The listing builds one solid part. Answer for the finished solid, in the listing's coordinates (mm). Face numbers are marked on the shaded views. A direction names the side the tool comes from. Give positions to 0.01 mm unless a question says otherwise; leave off trailing zeros. Write each loop counter-clockwise with the first axis right and the second up, starting at its lowest first coordinate (ties: lowest second). Pieces come first, ordered by that corner, then holes. Notation, with made-up numbers: (5, 45) -> (42, 45) arc R14 ccw to (42, 69) -> close; hole circle Ø11 at (-9.75, -7). An arc over 180 degrees is marked (long way). Put each result on its own line as item: value. Start each with the question number.
1) For a pull along X with two mould halves and no side action, classify the marked faces 1, 2 and 3 as released by +X, released by -X, zero draft, split by the parting line, or undercut.
2) For the marked faces 4, 5 and 6, determine the directions among +Z, -Z, +X, -X, +Y, -Y from which every point of the face is accessible in a straight line to the end or side of a thin tool.
3) Flat-ended cylindrical pins translate along their axes: pin 1 Ø6 at (x, y) = (8, 9.5) entering from +Z; pin 2 Ø6 at (x, z) = (-10.5, -39.5) entering from -Y; pin 3 Ø0.5 at (x, z) = (17.5, -27.5) entering from +Y; pin 4 Ø1 at (y, z) = (-5, -33) entering from -X. Find the tip coordinate at first contact, or state that the pin passes through.
4) Find the intervals of material crossed by line 1 along X through (y, z) = (11, -28.75); line 2 along Z through (x, y) = (7.5, -15.5); line 3 along Z through (x, y) = (-4.5, -20.5), in increasing order. Write a range as from..to.
5) A cutting plane is placed at A-A (z = -36.75). Write down the section's boundary in (x, y), then the cut area to 3 significant figures.
from build123d import *

# Parameters (mm, degrees)
CYLINDER101_R               = 0.8
CYLINDER101_DEPTH           = 5
BOX013_W                    = 2
BOX013_H                    = 5.5
BOX013_DEPTH                = 5
BOX012_W                    = 0.75
BOX012_H                    = 8
BOX012_DEPTH                = 5
CYLINDER100_R               = 3
CYLINDER100_DEPTH           = 5
CUT064_PLACEMENT_ANGLE      = 120
CYLINDER104_R               = 0.8
CYLINDER104_DEPTH           = 5
CUT067_PLACEMENT_ANGLE      = 60
CYLINDER102_R               = 0.8
CYLINDER102_DEPTH           = 5
CUT065_PLACEMENT_ANGLE      = 180
CYLINDER106_R               = 0.8
CYLINDER106_DEPTH           = 5
CYLINDER103_R               = 0.8
CYLINDER103_DEPTH           = 5
CUT066_PLACEMENT_ANGLE      = 240
CYLINDER098_R               = 0.8
CYLINDER098_DEPTH           = 5
CUT063_PLACEMENT_ANGLE      = 60
CYLINDER007_R               = 19.25
CYLINDER007_DEPTH           = 5
CYLINDER018_R               = 22.5
CYLINDER018_DEPTH           = 0.5
CYLINDER070_R               = 20
CYLINDER070_DEPTH           = 5
CYLINDER006_R               = 18.5
CYLINDER006_DEPTH           = 20
CYLINDER002_R               = 22.1
CYLINDER002_DEPTH           = 17
CYLINDER001_R               = 23.5
CYLINDER001_DEPTH           = 17
CYLINDER_R                  = 23.5
CYLINDER_DEPTH              = 20
CYLINDER003_R               = 22
CYLINDER003_DEPTH           = 17
CYLINDER004_R               = 23.5
CYLINDER004_DEPTH           = 10
CUT060_PLACEMENT_ANGLE      = 180
FUSION050_PLACEMENT_ANGLE   = 180
CYLINDER073_R               = 1
CYLINDER073_DEPTH           = 10
CYLINDER073_PLACEMENT_ANGLE = 120
CYLINDER075_R               = 1
CYLINDER075_DEPTH           = 10
CYLINDER075_PLACEMENT_ANGLE = 240
CYLINDER072_R               = 1
CYLINDER072_DEPTH           = 10
CYLINDER072_PLACEMENT_ANGLE = 60
CYLINDER074_R               = 1
CYLINDER074_DEPTH           = 10
CYLINDER076_R               = 1
CYLINDER076_DEPTH           = 10
CYLINDER076_PLACEMENT_ANGLE = 60
CYLINDER071_R               = 1
CYLINDER071_DEPTH           = 10
FUSION030_PLACEMENT_ANGLE   = 30


with BuildPart() as cylinder101:
    # Cylinder101 → Cylinder101 (new body)
    with BuildSketch(Plane(origin=(15.5, 0, 15), x_dir=(1, 0, 0), z_dir=(0, 0, 1))):
        Circle(CYLINDER101_R)
    extrude(amount=CYLINDER101_DEPTH)


with BuildPart() as cube013:
    # Box013 → Box013 (new body)
    with BuildSketch(Plane(origin=(16.5, -2.75, 15), x_dir=(1, 0, 0), z_dir=(0, 0, 1))):
        with Locations((1, 2.75)):
            Rectangle(BOX013_W, BOX013_H)
    extrude(amount=BOX013_DEPTH)


with BuildPart() as cube012:
    # Box012 → Box012 (new body)
    with BuildSketch(Plane(origin=(18.2, -4, 15), x_dir=(1, 0, 0), z_dir=(0, 0, 1))):
        with Locations((0.375, 4)):
            Rectangle(BOX012_W, BOX012_H)
    extrude(amount=BOX012_DEPTH)


with BuildPart() as cylinder100:
    # Cylinder100 → Cylinder100 (new body)
    with BuildSketch(Plane(origin=(15.5, 0, 15), x_dir=(1, 0, 0), z_dir=(0, 0, 1))):
        Circle(CYLINDER100_R)
    extrude(amount=CYLINDER100_DEPTH)


with BuildPart() as cut064:
    # Fusion043 base: copy of Cylinder100
    add(cylinder100.part)

    # Fusion043: union Cube013, Cube012
    add(cube013.part)
    add(cube012.part)

    # Cut064: cut Cylinder101
    add(cylinder101.part, mode=Mode.SUBTRACT)


with BuildPart() as cut064_1:
    # Cut064 placement: moved
    add(cut064.part.moved(Location((0, 0, 9))).rotate(Axis((0, 0, 9), (0, 0, 1)), CUT064_PLACEMENT_ANGLE))


with BuildPart() as cylinder104:
    # Cylinder104 → Cylinder104 (new body)
    with BuildSketch(Plane(origin=(15.5, 0, 15), x_dir=(1, 0, 0), z_dir=(0, 0, 1))):
        Circle(CYLINDER104_R)
    extrude(amount=CYLINDER104_DEPTH)


with BuildPart() as cut067:
    # Fusion046 base: copy of Cylinder100
    add(cylinder100.part)

    # Fusion046: union Cube013, Cube012
    add(cube013.part)
    add(cube012.part)

    # Cut067: cut Cylinder104
    add(cylinder104.part, mode=Mode.SUBTRACT)


with BuildPart() as cut067_1:
    # Cut067 placement: moved
    add(cut067.part.moved(Location((0, 0, 9))).rotate(Axis((0, 0, 9), (0, 0, -1)), CUT067_PLACEMENT_ANGLE))


with BuildPart() as cylinder102:
    # Cylinder102 → Cylinder102 (new body)
    with BuildSketch(Plane(origin=(15.5, 0, 15), x_dir=(1, 0, 0), z_dir=(0, 0, 1))):
        Circle(CYLINDER102_R)
    extrude(amount=CYLINDER102_DEPTH)


with BuildPart() as cut065:
    # Fusion044 base: copy of Cylinder100
    add(cylinder100.part)

    # Fusion044: union Cube013, Cube012
    add(cube013.part)
    add(cube012.part)

    # Cut065: cut Cylinder102
    add(cylinder102.part, mode=Mode.SUBTRACT)


with BuildPart() as cut065_1:
    # Cut065 placement: moved
    add(cut065.part.moved(Location((0, 0, 9))).rotate(Axis((0, 0, 9), (0, 0, 1)), CUT065_PLACEMENT_ANGLE))


with BuildPart() as cylinder106:
    # Cylinder106 → Cylinder106 (new body)
    with BuildSketch(Plane(origin=(15.5, 0, 15), x_dir=(1, 0, 0), z_dir=(0, 0, 1))):
        Circle(CYLINDER106_R)
    extrude(amount=CYLINDER106_DEPTH)


with BuildPart() as cut069:
    # Fusion048 base: copy of Cylinder100
    add(cylinder100.part)

    # Fusion048: union Cube013, Cube012
    add(cube013.part)
    add(cube012.part)

    # Cut069: cut Cylinder106
    add(cylinder106.part, mode=Mode.SUBTRACT)


with BuildPart() as cut069_1:
    # Cut069 placement: moved
    add(cut069.part.moved(Location((0, 0, 9))))


with BuildPart() as cylinder103:
    # Cylinder103 → Cylinder103 (new body)
    with BuildSketch(Plane(origin=(15.5, 0, 15), x_dir=(1, 0, 0), z_dir=(0, 0, 1))):
        Circle(CYLINDER103_R)
    extrude(amount=CYLINDER103_DEPTH)


with BuildPart() as cut066:
    # Fusion045 base: copy of Cylinder100
    add(cylinder100.part)

    # Fusion045: union Cube013, Cube012
    add(cube013.part)
    add(cube012.part)

    # Cut066: cut Cylinder103
    add(cylinder103.part, mode=Mode.SUBTRACT)


with BuildPart() as cut066_1:
    # Cut066 placement: moved
    add(cut066.part.moved(Location((0, 0, 9))).rotate(Axis((0, 0, 9), (0, 0, 1)), CUT066_PLACEMENT_ANGLE))


with BuildPart() as cylinder098:
    # Cylinder098 → Cylinder098 (new body)
    with BuildSketch(Plane(origin=(15.5, 0, 15), x_dir=(1, 0, 0), z_dir=(0, 0, 1))):
        Circle(CYLINDER098_R)
    extrude(amount=CYLINDER098_DEPTH)


with BuildPart() as fusion049:
    # Fusion042 base: copy of Cylinder100
    add(cylinder100.part)

    # Fusion042: union Cube013, Cube012
    add(cube013.part)
    add(cube012.part)

    # Cut063: cut Cylinder098
    add(cylinder098.part, mode=Mode.SUBTRACT)


with BuildPart() as fusion049_1:
    # Cut063 placement: moved
    add(fusion049.part.moved(Location((0, 0, 9))).rotate(Axis((0, 0, 9), (0, 0, 1)), CUT063_PLACEMENT_ANGLE))

    # Fusion049: union Cut064, Cut067, Cut065, Cut069, Cut066
    add(cut064_1.part)
    add(cut067_1.part)
    add(cut065_1.part)
    add(cut069_1.part)
    add(cut066_1.part)


with BuildPart() as cylinder007:
    # Cylinder007 → Cylinder007 (new body)
    with BuildSketch(Plane.XY.offset(5)):
        Circle(CYLINDER007_R)
    extrude(amount=CYLINDER007_DEPTH)


with BuildPart() as cone:
    # Cone → Cone (revolve)
    with BuildSketch(Plane(origin=(0, 0, 5), x_dir=(1, 0, 0), z_dir=(0, -1, 0))):
        Polygon((0, 0), (20, 0), (12, 6), (0, 6), align=None)
    revolve(axis=Axis((0, 0, 5), (0, 0, 1)))


with BuildPart() as cylinder018:
    # Cylinder018 → Cylinder018 (new body)
    with BuildSketch(Plane.XY):
        Circle(CYLINDER018_R)
    extrude(amount=CYLINDER018_DEPTH)


with BuildPart() as cylinder070:
    # Cylinder070 → Cylinder070 (new body)
    with BuildSketch(Plane.XY):
        Circle(CYLINDER070_R)
    extrude(amount=CYLINDER070_DEPTH)


with BuildPart() as cylinder006:
    # Cylinder006 → Cylinder006 (new body)
    with BuildSketch(Plane.XY):
        Circle(CYLINDER006_R)
    extrude(amount=CYLINDER006_DEPTH)


with BuildPart() as cylinder002:
    # Cylinder002 → Cylinder002 (new body)
    with BuildSketch(Plane.XY):
        Circle(CYLINDER002_R)
    extrude(amount=CYLINDER002_DEPTH)


with BuildPart() as cut:
    # Cylinder001 → Cylinder001 (new body)
    with BuildSketch(Plane.XY):
        Circle(CYLINDER001_R)
    extrude(amount=CYLINDER001_DEPTH)

    # Cut: cut Cylinder002
    add(cylinder002.part, mode=Mode.SUBTRACT)


with BuildPart() as cut_1:
    # Cut placement: moved
    add(cut.part.moved(Location((0, 0, 1.5))))


with BuildPart() as cut001:
    # Cylinder → Cylinder (new body)
    with BuildSketch(Plane.XY):
        Circle(CYLINDER_R)
    extrude(amount=CYLINDER_DEPTH)

    # Cut001: cut Cut
    add(cut_1.part, mode=Mode.SUBTRACT)


with BuildPart() as cylinder003:
    # Cylinder003 → Cylinder003 (new body)
    with BuildSketch(Plane.XY):
        Circle(CYLINDER003_R)
    extrude(amount=CYLINDER003_DEPTH)


with BuildPart() as rim_inner_rear:
    # Cylinder004 → Cylinder004 (new body)
    with BuildSketch(Plane.XY.offset(0.5)):
        Circle(CYLINDER004_R)
    extrude(amount=CYLINDER004_DEPTH)

    # Cut002: cut Cylinder003
    add(cylinder003.part, mode=Mode.SUBTRACT)


with BuildPart() as rim_inner_rear_1:
    # Cut002 placement: moved
    add(rim_inner_rear.part.moved(Location((0, 0, 4.5))))

    # Fusion: union Cut001
    add(cut001.part)

    # Cut031: cut Cylinder006
    add(cylinder006.part, mode=Mode.SUBTRACT)

    # Cut057: cut Cylinder070
    add(cylinder070.part, mode=Mode.SUBTRACT)

    # Cut058: cut Cylinder018
    add(cylinder018.part, mode=Mode.SUBTRACT)

    # Cut059: cut Cone
    add(cone.part, mode=Mode.SUBTRACT)

    # Cut060: cut Cylinder007
    add(cylinder007.part, mode=Mode.SUBTRACT)


with BuildPart() as rim_inner_rear_2:
    # Cut060 placement: moved
    add(rim_inner_rear_1.part.moved(Location((0, 0, 44))).rotate(Axis((0, 0, 44), (0, 1, 0)), CUT060_PLACEMENT_ANGLE))

    # Fusion050: union Fusion049
    add(fusion049_1.part)


with BuildPart() as rim_inner_rear_3:
    # Fusion050 placement: moved
    add(rim_inner_rear_2.part.rotate(Axis((0, 0, 0), (0, 1, 0)), FUSION050_PLACEMENT_ANGLE))


with BuildPart() as cylinder073:
    # Cylinder073 → Cylinder073 (new body)
    with BuildSketch(Plane.XY):
        Circle(CYLINDER073_R)
    extrude(amount=CYLINDER073_DEPTH)


with BuildPart() as cylinder073_1:
    # Cylinder073 placement: moved
    add(cylinder073.part.moved(Location((-9.25, 16.02147, 5))).rotate(Axis((-9.25, 16.02147, 5), (0, 0, 1)), CYLINDER073_PLACEMENT_ANGLE))


with BuildPart() as cylinder075:
    # Cylinder075 → Cylinder075 (new body)
    with BuildSketch(Plane.XY):
        Circle(CYLINDER075_R)
    extrude(amount=CYLINDER075_DEPTH)


with BuildPart() as cylinder075_1:
    # Cylinder075 placement: moved
    add(cylinder075.part.moved(Location((-9.25, -16.02147, 5))).rotate(Axis((-9.25, -16.02147, 5), (0, 0, 1)), CYLINDER075_PLACEMENT_ANGLE))


with BuildPart() as cylinder072:
    # Cylinder072 → Cylinder072 (new body)
    with BuildSketch(Plane.XY):
        Circle(CYLINDER072_R)
    extrude(amount=CYLINDER072_DEPTH)


with BuildPart() as cylinder072_1:
    # Cylinder072 placement: moved
    add(cylinder072.part.moved(Location((9.25, 16.02147, 5))).rotate(Axis((9.25, 16.02147, 5), (0, 0, 1)), CYLINDER072_PLACEMENT_ANGLE))


with BuildPart() as cylinder074:
    # Cylinder074 → Cylinder074 (new body)
    with BuildSketch(Plane(origin=(-18.5, 0, 5), x_dir=(-1, 0, 0), z_dir=(0, 0, 1))):
        Circle(CYLINDER074_R)
    extrude(amount=CYLINDER074_DEPTH)


with BuildPart() as cylinder076:
    # Cylinder076 → Cylinder076 (new body)
    with BuildSketch(Plane.XY):
        Circle(CYLINDER076_R)
    extrude(amount=CYLINDER076_DEPTH)


with BuildPart() as cylinder076_1:
    # Cylinder076 placement: moved
    add(cylinder076.part.moved(Location((9.25, -16.02147, 5))).rotate(Axis((9.25, -16.02147, 5), (0, 0, -1)), CYLINDER076_PLACEMENT_ANGLE))


with BuildPart() as obj1:
    # Cylinder071 → Cylinder071 (new body)
    with BuildSketch(Plane(origin=(18.5, 0, 5), x_dir=(1, 0, 0), z_dir=(0, 0, 1))):
        Circle(CYLINDER071_R)
    extrude(amount=CYLINDER071_DEPTH)

    # Fusion030: union Cylinder073, Cylinder075, Cylinder072, Cylinder074, Cylinder076
    add(cylinder073_1.part)
    add(cylinder075_1.part)
    add(cylinder072_1.part)
    add(cylinder074.part)
    add(cylinder076_1.part)


with BuildPart() as obj1_1:
    # Fusion030 placement: moved
    add(obj1.part.moved(Location((0, 0, -39))).rotate(Axis((0, 0, -39), (0, 0, 1)), FUSION030_PLACEMENT_ANGLE))

    # Fusion070: union rim-inner-rear_
    add(rim_inner_rear_3.part)


solid = obj1_1.part
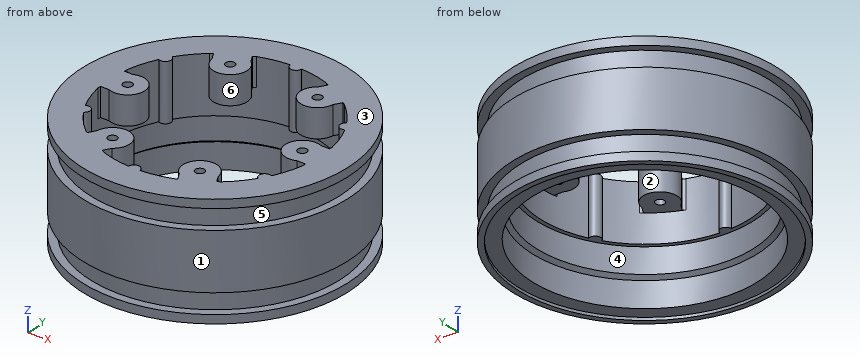
Reply:
1. face 1: split by the parting line
1. face 2: undercut
1. face 3: zero draft
2. face 4: -Z
2. face 5: none
2. face 6: +Z, -Z
3. pin 1: stops at z = -24
3. pin 2: stops at y = -22.26
3. pin 3: stops at y = 13.81
3. pin 4: stops at x = -23.07
4. line 1: x = -19.17..-14.87, -9.52..-5.98, 5.98..9.52, 14.87..19.17
4. line 2: z = -29..-24
4. line 3: z = -43.5..-24
5. outline: circle Ø47 at (0, 0); hole circle Ø38.5 at (0, 0)
5. area: 571 mm2
